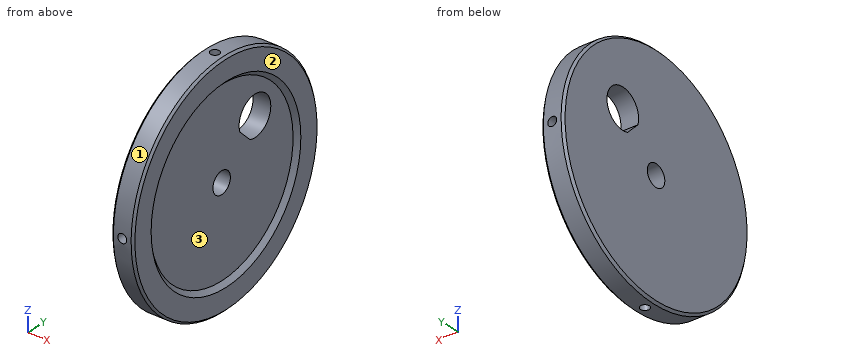
```python
from build123d import *

# Parameters (mm, degrees)
CUT_EXTRUDE1_DEPTH = 10
CIRPATTERN2_COUNT  = 4
CHAMFER1_SIZE      = 1
CHAMFER2_SIZE      = 1
SKETCH8_R          = 52.0992
CUT_EXTRUDE2_DEPTH = 0.0508


with BuildPart() as part:
    # Sketch1 → Revolve1 (revolve)
    with BuildSketch(Plane(origin=(0, 0, 0), x_dir=(1, 0, 0), z_dir=(0, 1, 0))):
        Polygon((0, 4.9022), (0, 52.0992), (10, 52.0992), (10, 42.0992), (8, 40.0992), (8, 4.9022), align=None)
    revolve(axis=Axis((0, 0, 0), (1, 0, 0)))

    # Sketch3 → Cut-Extrude1 (cut)
    with BuildSketch(Plane(origin=(8, 0, 0), x_dir=(0, 0, -1), z_dir=(1, 0, 0))):
        with BuildLine():
            Line((-16.012131778, 10.215581079), (-10.215581079, 16.012131778))
            ThreePointArc((-10.215581079, 16.012131778), (-14.077724842, 26.305561936), (-24.993250353, 24.993250353))
            ThreePointArc((-24.993250353, 24.993250353), (-26.305561936, 14.077724842), (-16.012131778, 10.215581079))
        make_face()
    extrude(amount=-CUT_EXTRUDE1_DEPTH, mode=Mode.SUBTRACT)

    # Sketch6 → #10-32 Tapped Hole1 (revolve, cut)
    with BuildSketch(Plane(origin=(5, 0, 52.0992), x_dir=(0, -1, 0), z_dir=(1, 0, 0))):
        Polygon((0, 0), (0, 9.713317848), (2.0193, 8.5), (2.0193, 0), align=None)
    f_10_32_tapped_hole1 = revolve(axis=Axis((5, 0, 58.4492), (0, 0, -1)), mode=Mode.SUBTRACT)

    # CirPattern2: #10-32 Tapped Hole1 ×4 about axis
    cirpattern2_axis = Axis((0, 0, 0), (-1, 0, 0))
    for i in range(1, CIRPATTERN2_COUNT):
        add(f_10_32_tapped_hole1.rotate(cirpattern2_axis, i * 360 / CIRPATTERN2_COUNT), mode=Mode.SUBTRACT)

    # Chamfer1
    chamfer1_edges = [part.edges().sort_by_distance(p)[0] for p in [
        (10, 0, 52.0992),
    ]]
    chamfer(chamfer1_edges, length=CHAMFER1_SIZE)

    # Chamfer2
    chamfer2_edges = [part.edges().sort_by_distance(p)[0] for p in [
        (0, 0, 52.0992),
    ]]
    chamfer(chamfer2_edges, length=CHAMFER2_SIZE)

    # Sketch8 → Cut-Extrude2 (cut)
    with BuildSketch(Plane(origin=(10, 0, 0), x_dir=(0, 0, -1), z_dir=(1, 0, 0))):
        Circle(SKETCH8_R)
    extrude(amount=-CUT_EXTRUDE2_DEPTH, mode=Mode.SUBTRACT)


solid = part.part
```
Read the model definition and answer for the solid it produces. Units are mm, in the model's axes. Face numbers are marked on the shaded views. Give positions to 0.01 mm unless a question says otherwise; leave off trailing zeros. Answer in a Markdown table with one row per item.
1) Each of these flat-tipped pins is pushed along its axis until it touches: pin 1 Ø1 at (x, z) = (8.5, 40) entering from +Y; pin 2 Ø4 at (x, z) = (7, -17) entering from -Y; pin 3 Ø24 at (y, z) = (-9, -13) entering from +X; pin 4 Ø4 at (y, z) = (-14.5, 37.5) entering from +X. Where does it stop, or does it pass through?
Results list:
| item | result |
|---|---|
| pin 1 | y = 33.97 |
| pin 2 | y = -49.89 |
| pin 3 | x = 8 |
| pin 4 | x = 9.95 |
2) Straight lines are drawn through the part: line 1 (X direction, y = 0, z = -48); line 2 (X direction, y = 3, z = -27); line 3 (Y direction, x = 8.5, z = -18). For each, find the intervals that lie inside material, in ascending order. Write a range as [from, to].
Results list:
| item | result |
|---|---|
| line 1 | [0, 2.98], [7.02, 9.95] |
| line 2 | [0, 8] |
| line 3 | [-48.89, -36.39], [36.39, 48.89] |
3) Determine the mould class of the marked faces 1, 2 and 3 for opening direction Y: released by +Y, released by -Y, zero draft, split by the parting line, or undercut.
Results list:
| item | result |
|---|---|
| face 1 | split by the parting line |
| face 2 | zero draft |
| face 3 | undercut |
